Drawing for the job (mm, zero at the part's lowest x, y, z). Give positions to 0.01 mm unless a question says otherwise; leave off trailing zeros. Order: outer loops, then holes, each group sorted by start corner. A loop starts at its lowest first (then second) coordinate and runs counter-clockwise, first axis right, second up. Notation, with made-up numbers: (7.5, -1.5) -> (49.5, -1.5) arc R34 cw to (49.5, 32.5) -> close; hole circle Ø8 at (-25, 18). An arc over 180 degrees is marked (long way). Use one line per item in the form item = value. Start each with the question number.
1) Drop a flat-ended pin along its axis: P1, Ø1, axis at y = 951, z = 10.5, coming from the +X side. Give the stop position or say it passes through.
2) Probe line 1 (X direction, y = 899.5, z = 5.5); line 2 (Y direction, x = 1005.5, z = 21); line 3 (Y direction, x = 866, z = 13.5). List the from-to ranges inside material, lowest first.
3) Cut at A-A, the plane z = 29.5. Give the cut face in (x, y), and give its area (3 significant figures).
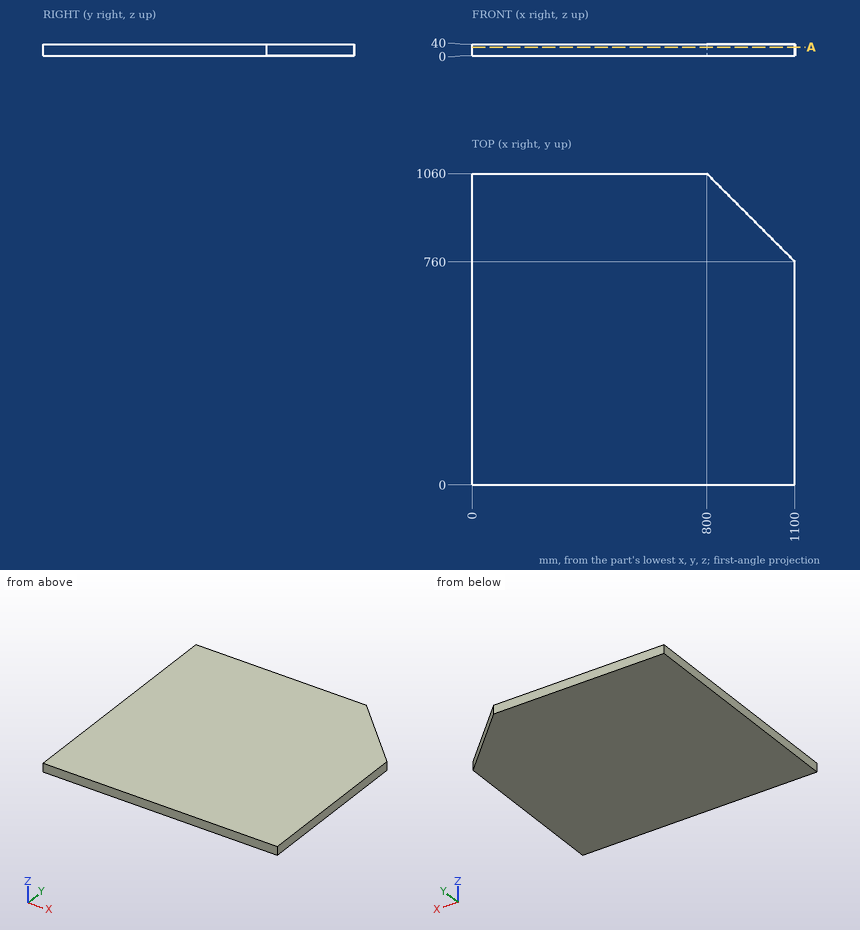
Result:
q1.P1 = 909.5
q2.line_1 = 0 to 960.5
q2.line_2 = 0 to 854.5
q2.line_3 = 0 to 994
q3.outline = (0, 0) -> (1100, 0) -> (1100, 760) -> (800, 1060) -> (0, 1060) -> close
q3.area = 1,120,000 mm²
